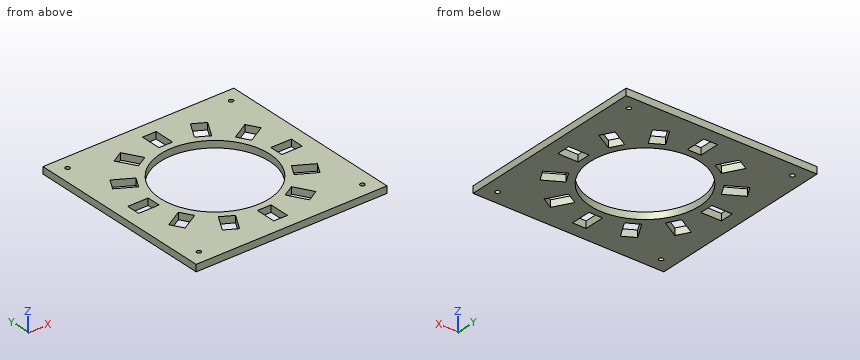
from build123d import *

# Parameters (mm, degrees)
F0_W      = 130
F0_H      = 5
F1_DEPTH  = 70
F2_W      = 140
F2_H      = 140
F3_DEPTH  = 5
F4_W      = 140
F4_H      = 140
F4_R      = 40
F5_DEPTH  = 5
F7_W      = 5
F7_H      = 15
F7_W_2    = 15
F7_H_2    = 5
F8_DEPTH  = 5
F9_W      = 140
F9_H      = 70
F10_DEPTH = 140
F11_R     = 1.6
F12_DEPTH = 5


with BuildPart() as f1:
    # F0 (on Top) → F1 (new body)
    with BuildSketch(Plane.XY):
        with Locations((0, 67.5)):
            Rectangle(F0_W, F0_H)
        Polygon((-65, -65), (-65, 65), (-65, 70), (-70, 70), (-70, -70), (-65, -70), align=None)
        Polygon((65, 70), (65, 65), (65, -65), (65, -70), (70, -70), (70, 70), align=None)
        with Locations((0, -67.5)):
            Rectangle(F0_W, F0_H)
    extrude(amount=F1_DEPTH)

    # F2 (on face) → F3 (join)
    with BuildSketch(Plane(origin=(0, 0, 0), x_dir=(1, 0, 0), z_dir=(0, 0, -1))):
        Rectangle(F2_W, F2_H)
    extrude(amount=-F3_DEPTH)

    # F4 (on face) → F5 (join)
    with BuildSketch(Plane.XY.offset(70)):
        Rectangle(F4_W, F4_H)
        Circle(F4_R, mode=Mode.SUBTRACT)
    extrude(amount=F5_DEPTH)

    # F7 (on face) → F8 (cut, through all)
    with BuildSketch(Plane.XY.offset(75)):
        Polygon((-41.471143, 18.169873), (-38.971143, 22.5), (-51.961524, 30), (-54.461524, 25.669873), align=None)
        Polygon((-51.961524, 30), (-38.971143, 22.5), (-36.471143, 26.830127), (-49.461524, 34.330127), align=None)
        with Locations((-2.5, 52.5)):
            Rectangle(F7_W, F7_H)
        with Locations((2.5, 52.5)):
            Rectangle(F7_W, F7_H)
        Polygon((51.961524, 30), (49.461524, 34.330127), (36.471143, 26.830127), (38.971143, 22.5), align=None)
        Polygon((54.461524, 25.669873), (51.961524, 30), (38.971143, 22.5), (41.471143, 18.169873), align=None)
        Polygon((-26.830127, 36.471143), (-22.5, 38.971143), (-30, 51.961524), (-34.330127, 49.461524), align=None)
        Polygon((-30, 51.961524), (-22.5, 38.971143), (-18.169873, 41.471143), (-25.669873, 54.461524), align=None)
        Polygon((51.961524, -30), (54.461524, -25.669873), (41.471143, -18.169873), (38.971143, -22.5), align=None)
        Polygon((49.461524, -34.330127), (51.961524, -30), (38.971143, -22.5), (36.471143, -26.830127), align=None)
        with Locations((-2.5, -52.5)):
            Rectangle(F7_W, F7_H)
        with Locations((2.5, -52.5)):
            Rectangle(F7_W, F7_H)
        Polygon((-51.961524, -30), (-49.461524, -34.330127), (-36.471143, -26.830127), (-38.971143, -22.5), align=None)
        Polygon((-54.461524, -25.669873), (-51.961524, -30), (-38.971143, -22.5), (-41.471143, -18.169873), align=None)
        Polygon((30, 51.961524), (25.669873, 54.461524), (18.169873, 41.471143), (22.5, 38.971143), align=None)
        Polygon((34.330127, 49.461524), (30, 51.961524), (22.5, 38.971143), (26.830127, 36.471143), align=None)
        with Locations((52.5, 2.5)):
            Rectangle(F7_W_2, F7_H_2)
        with Locations((52.5, -2.5)):
            Rectangle(F7_W_2, F7_H_2)
        Polygon((30, -51.961524), (34.330127, -49.461524), (26.830127, -36.471143), (22.5, -38.971143), align=None)
        Polygon((25.669873, -54.461524), (30, -51.961524), (22.5, -38.971143), (18.169873, -41.471143), align=None)
        Polygon((-26.830127, -36.471143), (-34.330127, -49.461524), (-30, -51.961524), (-22.5, -38.971143), align=None)
        Polygon((-22.5, -38.971143), (-30, -51.961524), (-25.669873, -54.461524), (-18.169873, -41.471143), align=None)
        with Locations((-52.5, 2.5)):
            Rectangle(F7_W_2, F7_H_2)
        with Locations((-52.5, -2.5)):
            Rectangle(F7_W_2, F7_H_2)
    extrude(amount=-F8_DEPTH, mode=Mode.SUBTRACT)

    # F9 (on face) → F10 (cut, through all)
    with BuildSketch(Plane.XZ.offset(70)):
        with Locations((0, 35)):
            Rectangle(F9_W, F9_H)
    extrude(amount=-F10_DEPTH, mode=Mode.SUBTRACT)

    # F11 (on face) → F12 (cut, through all)
    with BuildSketch(Plane.XY.offset(75)):
        with Locations((-60, -60)):
            Circle(F11_R)
        with Locations((-60, 60)):
            Circle(F11_R)
        with Locations((60, -60)):
            Circle(F11_R)
        with Locations((60, 60)):
            Circle(F11_R)
    extrude(amount=-F12_DEPTH, mode=Mode.SUBTRACT)


solid = f1.part
Geometry check sheet. Reference: the model listing, model coordinates, mm. Round coordinates to 2 decimals unless told otherwise and drop trailing zeros. Write each loop counter-clockwise with the first axis right and the second up, starting at its lowest first coordinate (ties: lowest second). Pieces come first, ordered by that corner, then holes.
Item 1: Material ranges on line 1 along Y through (x, z) = (0, 70.95); line 2 along X through (y, z) = (30, 74.05); line 3 along X through (y, z) = (43.5, 74.6), recorded low to high.
Determined:
line 1: y = -70 to -60, -45 to -40, 40 to 45, 60 to 70
line 2: x = -70 to -51.96, -41.96 to -26.46, 26.46 to 41.96, 51.96 to 70
line 3: x = -70 to -30.89, -19.34 to 19.34, 30.89 to 70
Item 2: Section check C-C (z = 74.15). Give the number of separate pieces and of enclosed holes in the cut face, plus the area to 3 significant figures.
Determined:
separate pieces: 1
enclosed holes: 17
area: 12,700 mm2
Item 3: Section check A-A (x = 0). Record the boundary of the cut face in (y, z).
Determined:
outline: (-70, 70) - (-60, 70) - (-60, 75) - (-70, 75) - close; (-45, 70) - (-40, 70) - (-40, 75) - (-45, 75) - close; (40, 70) - (45, 70) - (45, 75) - (40, 75) - close; (60, 70) - (70, 70) - (70, 75) - (60, 75) - close
